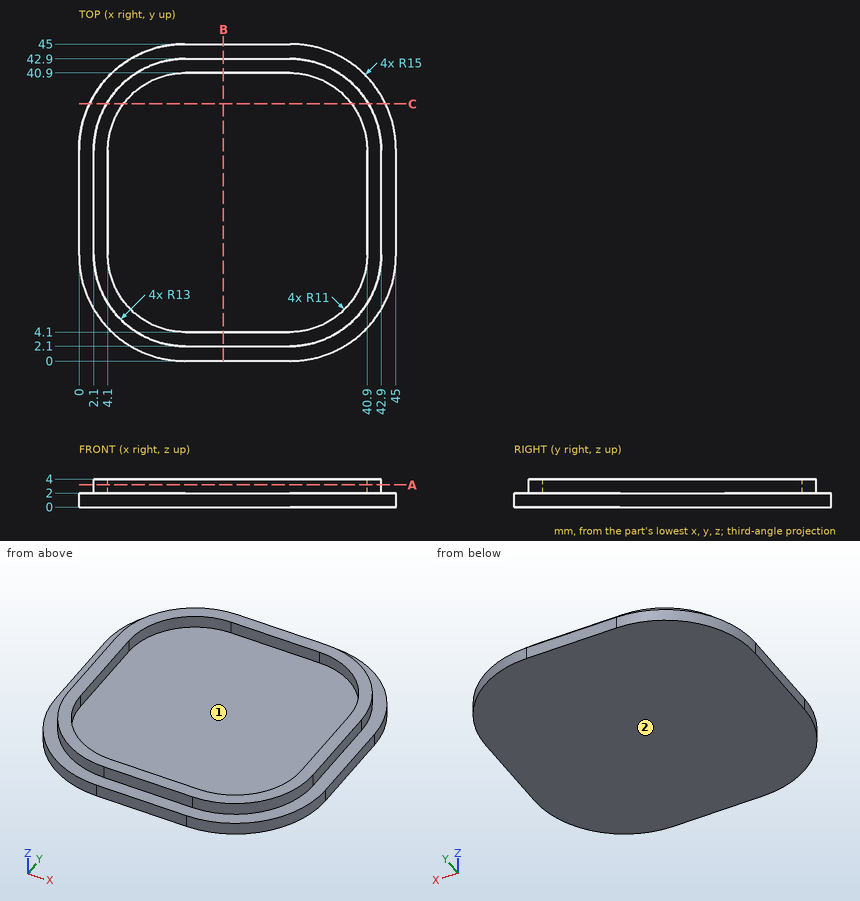
Can you work these out from the drawing? Everything is in mm from the part's minimum corner. Round coordinates to 2 decimals unless told otherwise and drop trailing zeros. Order: outer loops, then holes, each group sorted by start corner. A loop starts at its lowest first (then second) coordinate and runs counter-clockwise, first axis right, second up.
(1) If we section it at A-A (z = 3.15): Please give me the cut outline in (x, y).
Results are:
outline: (2.1, 15.1) arc R13 ccw to (15.1, 2.1) - (29.9, 2.1) arc R13 ccw to (42.9, 15.1) - (42.9, 29.9) arc R13 ccw to (29.9, 42.9) - (15.1, 42.9) arc R13 ccw to (2.1, 29.9) - close; hole (4.1, 15.1) arc R11 ccw to (15.1, 4.1) - (29.9, 4.1) arc R11 ccw to (40.9, 15.1) - (40.9, 29.9) arc R11 ccw to (29.9, 40.9) - (15.1, 40.9) arc R11 ccw to (4.1, 29.9) - close
(2) If I drill on L1, parallel to X at y = 16.5, z = 3; L2, parallel to Z at x = 33.5, y = 33; L3, parallel to Y at x = 11.5, z = 2.15, over which ranges is the centre line in solid material (lowest first)?
Results are:
L1: x = 2.1 to 4.1, 40.9 to 42.9
L2: z = 0 to 2
L3: y = 2.61 to 4.71, 40.29 to 42.39
(3) If we section it at C-C (y = 36.5): Please give me the cut outline in (x, z), plus the area to 3 significant figures.
Results are:
outline: (1.48, 0) - (43.52, 0) - (43.52, 2) - (41.1, 2) - (41.1, 4) - (38.7, 4) - (38.7, 2) - (6.3, 2) - (6.3, 4) - (3.9, 4) - (3.9, 2) - (1.48, 2) - close
area: 93.7 mm2
(4) I'm going to push flat-ended pins straight in: pin 1 (1.6 mm diameter, centred on y = 22, z = 3, fed in from -X); pin 2 (1 mm diameter, centred on x = 24.5, z = 3.5, fed in from -Y); pin 3 (1.5 mm diameter, centred on x = 11, z = 1.5, fed in from +Y). Where does each tip first touch, or does it pass through?
Results are:
pin 1: stops at x = 2.1
pin 2: stops at y = 2.1
pin 3: stops at y = 44.64
(5) We'd pull the mould along X, two halves only. Please class the marked faces 1 and 2: +X half, -X half, draft (parallel to the pull), parting line (faces both ways), or undercut.
Results are:
face 1: undercut
face 2: draft
(6) If we section it at B-B (x = 20.5): Please give me the cut outline in (y, z), plus the area to 3 significant figures.
Results are:
outline: (0, 0) - (45, 0) - (45, 2) - (42.9, 2) - (42.9, 4) - (40.9, 4) - (40.9, 2) - (4.1, 2) - (4.1, 4) - (2.1, 4) - (2.1, 2) - (0, 2) - close
area: 98.0 mm2
